```python
from build123d import *

# Parameters (mm, degrees)
SKETCH1_W           = 150
SKETCH1_H           = 250
SKETCH1_R           = 2.05
SKETCH1_R_2         = 1.25
SKETCH1_W_2         = 40.2
SKETCH1_H_2         = 20.4
BOSS_EXTRUDE1_DEPTH = 6.35
FILLET1_R           = 16


with BuildPart() as part:
    # Sketch1 → Boss-Extrude1 (new body)
    with BuildSketch(Plane(origin=(0, 0, 0), x_dir=(1, 0, 0), z_dir=(0, 1, 0))):
        Rectangle(SKETCH1_W, SKETCH1_H)
        with Locations(Location((-71, 5, 0), (0, 0, 270))):
            Circle(SKETCH1_R, mode=Mode.SUBTRACT)
        with Locations(Location((-71, -5, 0), (0, 0, 270))):
            Circle(SKETCH1_R, mode=Mode.SUBTRACT)
        with Locations(Location((-71, -100, 0), (0, 0, 270))):
            Circle(SKETCH1_R, mode=Mode.SUBTRACT)
        with Locations(Location((-71, -110, 0), (0, 0, 270))):
            Circle(SKETCH1_R, mode=Mode.SUBTRACT)
        with Locations(Location((-71, 110, 0), (0, 0, 90))):
            Circle(SKETCH1_R, mode=Mode.SUBTRACT)
        with Locations(Location((-71, 100, 0), (0, 0, 90))):
            Circle(SKETCH1_R, mode=Mode.SUBTRACT)
        with Locations(Location((-21.4, 100, 0), (0, 0, 270))):
            Circle(SKETCH1_R, mode=Mode.SUBTRACT)
        with Locations(Location((-21.4, 110, 0), (0, 0, 270))):
            Circle(SKETCH1_R, mode=Mode.SUBTRACT)
        with Locations(Location((-21.4, -110, 0), (0, 0, 90))):
            Circle(SKETCH1_R, mode=Mode.SUBTRACT)
        with Locations(Location((-21.4, -100, 0), (0, 0, 90))):
            Circle(SKETCH1_R, mode=Mode.SUBTRACT)
        with Locations(Location((-21.4, -5, 0), (0, 0, 90))):
            Circle(SKETCH1_R, mode=Mode.SUBTRACT)
        with Locations(Location((-21.4, 5, 0), (0, 0, 90))):
            Circle(SKETCH1_R, mode=Mode.SUBTRACT)
        with Locations(Location((21.4, 5, 0), (0, 0, 270))):
            Circle(SKETCH1_R, mode=Mode.SUBTRACT)
        with Locations(Location((21.4, -5, 0), (0, 0, 270))):
            Circle(SKETCH1_R, mode=Mode.SUBTRACT)
        with Locations(Location((21.4, -100, 0), (0, 0, 270))):
            Circle(SKETCH1_R, mode=Mode.SUBTRACT)
        with Locations(Location((21.4, -110, 0), (0, 0, 270))):
            Circle(SKETCH1_R, mode=Mode.SUBTRACT)
        with Locations(Location((21.4, 110, 0), (0, 0, 90))):
            Circle(SKETCH1_R, mode=Mode.SUBTRACT)
        with Locations(Location((21.4, 100, 0), (0, 0, 90))):
            Circle(SKETCH1_R, mode=Mode.SUBTRACT)
        with Locations(Location((71, 100, 0), (0, 0, 270))):
            Circle(SKETCH1_R, mode=Mode.SUBTRACT)
        with Locations(Location((71, 110, 0), (0, 0, 270))):
            Circle(SKETCH1_R, mode=Mode.SUBTRACT)
        with Locations(Location((71, -110, 0), (0, 0, 90))):
            Circle(SKETCH1_R, mode=Mode.SUBTRACT)
        with Locations(Location((71, -100, 0), (0, 0, 90))):
            Circle(SKETCH1_R, mode=Mode.SUBTRACT)
        with Locations(Location((71, -5, 0), (0, 0, 90))):
            Circle(SKETCH1_R, mode=Mode.SUBTRACT)
        with Locations(Location((71, 5, 0), (0, 0, 90))):
            Circle(SKETCH1_R, mode=Mode.SUBTRACT)
        with Locations(Location((-40.75, -22, 0), (0, 0, 270))):
            Circle(SKETCH1_R_2, mode=Mode.SUBTRACT)
        with Locations(Location((-40.75, -71, 0), (0, 0, 270))):
            Circle(SKETCH1_R_2, mode=Mode.SUBTRACT)
        with Locations(Location((17.25, -71, 0), (0, 0, 270))):
            Circle(SKETCH1_R_2, mode=Mode.SUBTRACT)
        with Locations(Location((17.25, -22, 0), (0, 0, 270))):
            Circle(SKETCH1_R_2, mode=Mode.SUBTRACT)
        with Locations(Location((-53, 40, 0), (0, 0, 270))):
            Circle(SKETCH1_R, mode=Mode.SUBTRACT)
        with Locations(Location((-10, 40, 0), (0, 0, 270))):
            Circle(SKETCH1_R, mode=Mode.SUBTRACT)
        with Locations(Location((10, 40, 0), (0, 0, 90))):
            Circle(SKETCH1_R, mode=Mode.SUBTRACT)
        with Locations(Location((53, 40, 0), (0, 0, 90))):
            Circle(SKETCH1_R, mode=Mode.SUBTRACT)
        with Locations((-46.2, -105)):
            Rectangle(SKETCH1_W_2, SKETCH1_H_2, mode=Mode.SUBTRACT)
        with Locations((46.2, -105)):
            Rectangle(SKETCH1_W_2, SKETCH1_H_2, mode=Mode.SUBTRACT)
        with Locations((-46.2, 105)):
            Rectangle(SKETCH1_W_2, SKETCH1_H_2, mode=Mode.SUBTRACT)
        with Locations((46.2, 105)):
            Rectangle(SKETCH1_W_2, SKETCH1_H_2, mode=Mode.SUBTRACT)
        with Locations((-46.2, 0)):
            Rectangle(SKETCH1_W_2, SKETCH1_H_2, mode=Mode.SUBTRACT)
        with Locations((46.2, 0)):
            Rectangle(SKETCH1_W_2, SKETCH1_H_2, mode=Mode.SUBTRACT)
    extrude(amount=BOSS_EXTRUDE1_DEPTH)

    # Fillet1
    fillet1_edges = [part.edges().sort_by_distance(p)[0] for p in [
        (75, 3.175, 125),
        (-75, 3.175, 125),
        (-75, 3.175, -125),
        (75, 3.175, -125),
    ]]
    fillet(fillet1_edges, radius=FILLET1_R)


solid = part.part
```
Design review of the part built by this model. Coordinates are the model's own, in mm. A direction names the side the tool comes from. Give positions to 0.01 mm unless a question says otherwise; leave off trailing zeros. Write each loop counter-clockwise with the first axis right and the second up, starting at its lowest first coordinate (ties: lowest second). Pieces come first, ordered by that corner, then holes. Notation, with made-up numbers: (15, 11.25) -> (29, 11.25) arc R18 cw to (29, 17.25) -> close; hole circle Ø4 at (4, -16). An arc over 180 degrees is marked (long way). Answer in a Markdown table with one row per item.
(1) To check wall thickness, follow probe 1 along Z at (x, y) = (32, 2.75); probe 2 along X at (y, z) = (4.25, 106.5); probe 3 along Z at (x, y) = (-63, 0.5). State the ranges of each line that lie inside material, in increasing order.
Results:
| item | result |
|---|---|
| probe 1 | -125 to -115.2, -94.8 to -10.2, 10.2 to 94.8, 115.2 to 125 |
| probe 2 | -75 to -66.3, -26.1 to 26.1, 66.3 to 75 |
| probe 3 | -124.49 to -115.2, -94.8 to -10.2, 10.2 to 94.8, 115.2 to 124.49 |
(2) Mouldability with a two-part tool opening along X and no side actions: class faces 1 (the cylindrical face through (70.189, 3.219, 120.437)), 2 (the flat face through (-46, 3, -10.2)), 3 (the flat face through (-46, 3, -94.8)), 4 (the cylindrical face through (-70.437, 3.219, 120.189)) as +X half, -X half, draft (parallel to the pull), parting line (faces both ways), or undercut.
Results:
| item | result |
|---|---|
| face 1 | +X half |
| face 2 | undercut |
| face 3 | undercut |
| face 4 | -X half |
(3) Consider section B-B (y = 3). Count the separate pieces of the cut face and the enclosed holes in it, then the cut area to 3 significant figures.
Results:
| item | result |
|---|---|
| separate pieces | 1 |
| enclosed holes | 38 |
| area | 32,000 mm2 |
(4) Consider section A-A (x = 36). State the section outline as (y, z) points, then the cut area to 3 significant figures.
Results:
| item | result |
|---|---|
| outline | (0, -125) -> (6.35, -125) -> (6.35, -115.2) -> (0, -115.2) -> close; (0, -94.8) -> (6.35, -94.8) -> (6.35, -10.2) -> (0, -10.2) -> close; (0, 10.2) -> (6.35, 10.2) -> (6.35, 94.8) -> (0, 94.8) -> close; (0, 115.2) -> (6.35, 115.2) -> (6.35, 125) -> (0, 125) -> close |
| area | 1,200 mm2 |
(5) For faces 5 (the flat face through (-1, 6.35, -2)), 6 (the flat face through (46, 3, -94.8)), list the 3-axis set-ups (+Z, -Z, +X, -X, +Y, -Y) from which the entire face can be reached by the end or side of a thin tool; tool diameter is ignored.
Results:
| item | result |
|---|---|
| face 5 | +Z, -Z, +X, -X, +Y |
| face 6 | +Y, -Y |
